Part model, mm, in its own coordinate system. A direction names the side the tool comes from. Round coordinates to 2 decimals unless told otherwise and drop trailing zeros. Write each loop counter-clockwise with the first axis right and the second up, starting at its lowest first coordinate (ties: lowest second). Pieces come first, ordered by that corner, then holes. Notation, with made-up numbers: M 74,54 L 131,54 A18 cw 131,76 Z; hole C 56.5,-24.5 d8. An arc over 180 degrees is marked long. Answer as a JSON object with one key per item and string values. Group by question number.
1. Which spindle directions (+Z, -Z, +X, -X, +Y, -Y) get a long thin tool onto all of the face, cutting with end or side? Do faces 3 (the face through (-4, 0, -2)), 4 (the face through (232.16, 3.13, 15.14)). Say none if no direction does.
2. Band-saw the part on B-B, the plane x = 80. Write the cut outline in (y, z), plus the area to 3 significant figures.
3. Band-saw the part on A-A, the plane y = 3.75. Count the separate pieces of the cut face and the enclosed holes in it, plus the area to 3 significant figures.
4. Two-plate mould, pull along X, no slides. Class faces 1 (the face through (80.29, 3.13, 15.14)), 2 (the face through (-4, 6.35, -2)): +X half, -X half, draft (parallel to the pull), parting line (faces both ways), or undercut.
5. Drill centre lines: line 1 (Z direction, x = 254.4, y = 4.25); line 2 (X direction, y = 3.5, z = 102.5); line 3 (X direction, y = 4.5, z = 42.5) (3 decimals). Where is each one in solid material? Low to high. Write a range as from..to.
from build123d import *

# Parameters (mm, degrees)
SKETCH1_W           = 558.8
SKETCH1_H           = 225
BOSS_EXTRUDE1_DEPTH = 6.35
SKETCH2_W           = 166.35
SKETCH2_H           = 143.7
CUT_EXTRUDE1_DEPTH  = 7.35
FILLET1_R           = 25.4
SKETCH3_R           = 3.2
CUT_EXTRUDE2_DEPTH  = 7.35


with BuildPart() as part:
    # Sketch1 → Boss-Extrude1 (new body)
    with BuildSketch(Plane(origin=(0, 0, 0), x_dir=(1, 0, 0), z_dir=(0, 1, 0))):
        Rectangle(SKETCH1_W, SKETCH1_H)
    extrude(amount=BOSS_EXTRUDE1_DEPTH)

    # Sketch2 → Cut-Extrude1 (cut, through all)
    with BuildSketch(Plane(origin=(0, 6.35, 0), x_dir=(1, 0, 0), z_dir=(0, 1, 0))):
        with Locations((156.225, -79.35)):
            Rectangle(SKETCH2_W, SKETCH2_H)
    extrude(amount=-CUT_EXTRUDE1_DEPTH, mode=Mode.SUBTRACT)

    # Fillet1
    fillet1_edges = [part.edges().sort_by_distance(p)[0] for p in [
        (239.4, 3.175, 7.5),
        (73.05, 3.175, 7.5),
    ]]
    fillet(fillet1_edges, radius=FILLET1_R)

    # Sketch3 → Cut-Extrude2 (cut, through all)
    with BuildSketch(Plane(origin=(0, 6.35, 0), x_dir=(1, 0, 0), z_dir=(0, 1, 0))):
        with Locations((-265.017168878, -102.5)):
            Circle(SKETCH3_R)
        with Locations((-265.017168878, -47.5)):
            Circle(SKETCH3_R)
        with Locations((-25.017168878, -47.5)):
            Circle(SKETCH3_R)
        with Locations((-25.017168878, -102.5)):
            Circle(SKETCH3_R)
        with Locations((101.644095195, 75)):
            Circle(SKETCH3_R)
        with Locations((149.275492403, 102.5)):
            Circle(SKETCH3_R)
        with Locations((149.275492403, 47.5)):
            Circle(SKETCH3_R)
        with Locations((254.4, 92.5)):
            Circle(SKETCH3_R)
        with Locations((254.4, 42.5)):
            Circle(SKETCH3_R)
        with Locations((254.4, -42.5)):
            Circle(SKETCH3_R)
        with Locations((254.4, -92.5)):
            Circle(SKETCH3_R)
        with Locations((34.575, -42.5)):
            Circle(SKETCH3_R)
        with Locations((34.575, -92.5)):
            Circle(SKETCH3_R)
    extrude(amount=-CUT_EXTRUDE2_DEPTH, mode=Mode.SUBTRACT)


solid = part.part
Worked answers:
{
 "1": {"face 3": "+Z, -Z, +X, -X, -Y", "face 4": "+Z, +Y, -Y"},
 "2": {"outline": "M 0,-112.5 L 6.35,-112.5 L 6.35,15.44 L 0,15.44 Z", "area": "812 mm^2"},
 "3": {"separate pieces": "1", "enclosed holes": "13", "area": "108,000 mm^2"},
 "4": {"face 1": "undercut", "face 2": "draft"},
 "5": {"line 1": "z = -112.5..-95.7, -89.3..-45.7, -39.3..39.3, 45.7..89.3, 95.7..112.5", "line 2": "x = -279.4..-268.22, -261.82..-28.22, -21.82..73.05, 239.4..279.4", "line 3": "x = -279.4..31.375, 37.775..73.05, 239.4..251.2, 257.6..279.4"}
}
